The model under review builds one solid part; all positions refer to its coordinate system, in mm. Coordinates: 2 decimals unless noted, no trailing zeros. Write each loop counter-clockwise with the first axis right and the second up, starting at its lowest first coordinate (ties: lowest second). Pieces come first, ordered by that corner, then holes.
1) For line 1 (Z direction, x = -10, y = -8.5); line 2 (Z direction, x = 0, y = -6); line 3 (X direction, y = -7, z = -2), list the stretches that pass through material, from the lowest coordinate up.
2) Add section C-C, the plane y = -8.5. State the section outline as (x, z) points.
3) Add section D-D, the plane z = 3.25. State the section outline as (x, y) points, then the cut area to 3 significant figures.
4) Add section B-B, the plane x = 0. State the section outline as (y, z) points, then the cut area to 3 significant figures.
5) Mouldability with a two-part tool opening along Z and no side actions: class faces 1 (the cylindrical face through (-12.5, -5.9, 0.1)), 2 (the flat face through (4, 0, -4)), 3 (the cylindrical face through (17, -6, 0)) as released by +Z, released by -Z, zero draft, split by the parting line, or undercut.
6) For P1, Ø4, axis at x = 0.5, z = -3.5, coming from the +Y side; P2, Ø4, axis at x = -2, z = 2, coming from the +Y side, all flat-tipped, find the tip position at first contact; note any pin that passes through.
7) Add section A-A, the plane z = 0. State the section outline as (x, y) points, then the cut area to 3 significant figures.
from build123d import *

# Parameters (mm, degrees)
F0_R     = 17
F0_R_2   = 2.5
F0_R_3   = 5
F1_DEPTH = 12
F3_DEPTH = 25


with BuildPart() as f1:
    # F0 (on Front) → F1 (new body)
    with BuildSketch(Plane.XZ):
        Circle(F0_R)
        with Locations((-10, 0)):
            Circle(F0_R_2, mode=Mode.SUBTRACT)
        Circle(F0_R_3, mode=Mode.SUBTRACT)
        with Locations((10, 0)):
            Circle(F0_R_2, mode=Mode.SUBTRACT)
    extrude(amount=F1_DEPTH)

    # F2 (on face) → F3 (cut)
    with BuildSketch(Plane(origin=(0, 0, 0), x_dir=(-1, 0, 0), z_dir=(0, 1, 0))):
        with BuildLine():
            ThreePointArc((14.2954538228, 9.2), (0, 17), (-14.2954538228, 9.2))
            Line((-14.2954538228, 9.2), (14.2954538228, 9.2))
        make_face()
        with BuildLine():
            Line((14.2954538228, -9.2), (-14.2954538228, -9.2))
            ThreePointArc((-14.2954538228, -9.2), (0, -17), (14.2954538228, -9.2))
        make_face()
    extrude(amount=-F3_DEPTH, mode=Mode.SUBTRACT)


solid = f1.part
Geometry results:
1. line 1: z = -9.2 to -2.5, 2.5 to 9.2
1. line 2: z = -9.2 to -5, 5 to 9.2
1. line 3: x = -16.88 to -11.5, -8.5 to -4.58, 4.58 to 8.5, 11.5 to 16.88
2. outline: (-14.3, -9.2) - (14.3, -9.2) arc R17 ccw to (14.3, 9.2) - (-14.3, 9.2) arc R17 ccw to start; hole circle Ø5 at (-10, 0); hole circle Ø10 at (0, 0); hole circle Ø5 at (10, 0)
3. outline: (-16.69, -12) - (-3.8, -12) - (-3.8, 0) - (-16.69, 0) - close; (3.8, -12) - (16.69, -12) - (16.69, 0) - (3.8, 0) - close
3. area: 309 mm2
4. outline: (-12, -9.2) - (0, -9.2) - (0, -5) - (-12, -5) - close; (-12, 5) - (0, 5) - (0, 9.2) - (-12, 9.2) - close
4. area: 101 mm2
5. face 1: undercut
5. face 2: zero draft
5. face 3: split by the parting line
6. P1: stops at y = 0
6. P2: passes through
7. outline: (-17, -12) - (-12.5, -12) - (-12.5, 0) - (-17, 0) - close; (-7.5, -12) - (-5, -12) - (-5, 0) - (-7.5, 0) - close; (5, -12) - (7.5, -12) - (7.5, 0) - (5, 0) - close; (12.5, -12) - (17, -12) - (17, 0) - (12.5, 0) - close
7. area: 168 mm2
